Solid Edge part; units mm, degrees
sketch "Sketch1" plane through (0, 0, 0) normal (0, 0, 1) x (1, 0, 0)
  circle A0 centre (0, 0) radius 2.5
  circle A1 centre (0, 0) radius 5
extrude "Protrusion1" add sketch "Sketch1" along normal blind 5
sketch "Sketch2" plane through (0, 0, 5) normal (0, 0, 1) x (1, 0, 0)
  line L0 (-4, 3) -> (4, 3)
  line L1 (4, 30) -> (4, 3)
  line L2 (-4, 30) -> (4, 30)
  line L3 (-4, 3) -> (-4, 30)
  dimension "D1" = 4
extrude "ExtrudedProtrusion_2" add sketch "Sketch2" against normal blind 3
sketch "Sketch3" plane through (0, 16.5, 2) normal (0, 0, -1) x (0, 1, 0)
  line L0 (13.5, 4) -> (13.5, -4)
  line L1 (13.5, -4) -> (5.5, -4)
  line L2 (5.5, -4) -> (5.5, 4)
  line L3 (5.5, 4) -> (13.5, 4)
  dimension "D1" = 5.5
extrude "ExtrudedProtrusion_3" add sketch "Sketch3" along normal blind 18.35
fillet "Round1" radius 3 2 edges at (0, 22, 2) (0, 30, 5)
properties material "Polyethylene, low density"
Source: CAD feature listing. Evaluate the final solid. Frame: model axes, mm. A direction names the side the tool comes from. Coordinates: 2 decimals unless noted, no trailing zeros. Loops run counter-clockwise (first coordinate to the right, second up) from the corner with the lowest first, then second, coordinate; pieces in that order, holes last. Notation, with made-up numbers: (49, -2) -> (81, -2) arc R26 ccw to (81, 18) -> close; hole circle Ø8 at (1, -7). An arc over 180 degrees is marked (long way). Answer in a Markdown table with one row per item. Add a question column.
Q1. Section D-D on x = 1.75. Return the cut outline in (y, z).
Q2. Ray query, line 1 along Y through (x, z) = (0, 2.15); line 2 along Y through (x, z) = (3.5, -12.25); line 3 along Z through (x, y) = (-0.25, -3.5). Return the intervals inside material, ascending.
Q3. Reachability of faces 4 (the face through (-4, 22.3, -3.2)), 5 (the face through (3, -4, 2)), 6 (the face through (0, 30, -7)), 7 (the face through (2, -2, 0)), 8 (the face through (4, 23, -3)) from +Z, -Z, +X, -X, +Y, -Y: full face, straight path, thin tool, end or side. Return the list, or none.
Q4. Contact query for flat-ended pins moving along their axis: pin 1 Ø2 at (x, y) = (-2.5, 20) entering from -Z; pin 2 Ø10.5 at (y, z) = (20.5, -3.5) entering from -X; pin 3 Ø4 at (x, z) = (1, -11) entering from -Y. Output: stop coordinate, or through.
Q5. Section B-B on y = 0. Return the cut outline in (x, z).
Q6. Section C-C on z = 0.75. Return the cut outline in (x, y).
Q7. Pull-direction query (Y, two-part tool) for faces 1 (the face through (0, 26, -16.35)), 2 (the face through (0.06, 21.14, 1.1)), 3 (the face through (0, 22, -9)); classes: pulls with the +Y half, pulls with the -Y half, needs draft (parallel to the pull), parting line crosses it, or undercut.
Q8. Section A-A on x = 0. Return the cut outline in (y, z), and give its area (3 significant figures).
Computed values:
| question | item | result |
|---|---|---|
| 1 | outline | (-4.68, 0) -> (-1.79, 0) -> (-1.79, 5) -> (-4.68, 5) -> close; (1.79, 0) -> (4.68, 0) -> (4.68, 2) -> (19, 2) arc R3 cw to (22, -1) -> (22, -16.35) -> (30, -16.35) -> (30, 2) arc R3 ccw to (27, 5) -> (1.79, 5) -> close |
| 2 | line 1 | y = -5 to -2.5, 2.5 to 30 |
| 2 | line 2 | y = 22 to 30 |
| 2 | line 3 | z = 0 to 5 |
| 3 | face 4 | +Z, -Z, -X, +Y |
| 3 | face 5 | -Z |
| 3 | face 6 | +Z, -Z, +X, -X, +Y |
| 3 | face 7 | -Z, +X, -X, -Y |
| 3 | face 8 | +Z, -Z, +X, +Y |
| 4 | pin 1 | stops at z = 1.24 |
| 4 | pin 2 | stops at x = -4 |
| 4 | pin 3 | stops at y = 22 |
| 5 | outline | (-5, 0) -> (-2.5, 0) -> (-2.5, 5) -> (-5, 5) -> close; (2.5, 0) -> (5, 0) -> (5, 5) -> (2.5, 5) -> close |
| 6 | outline | circle Ø10 at (0, 0); (-4, 21.44) -> (4, 21.44) -> (4, 30) -> (-4, 30) -> close; hole circle Ø5 at (0, 0) |
| 7 | face 1 | needs draft |
| 7 | face 2 | undercut |
| 7 | face 3 | pulls with the -Y half |
| 8 | outline | (-5, 0) -> (-2.5, 0) -> (-2.5, 5) -> (-5, 5) -> close; (2.5, 0) -> (5, 0) -> (5, 2) -> (19, 2) arc R3 cw to (22, -1) -> (22, -16.35) -> (30, -16.35) -> (30, 2) arc R3 ccw to (27, 5) -> (2.5, 5) -> close |
| 8 | area | 247 mm^2 |
